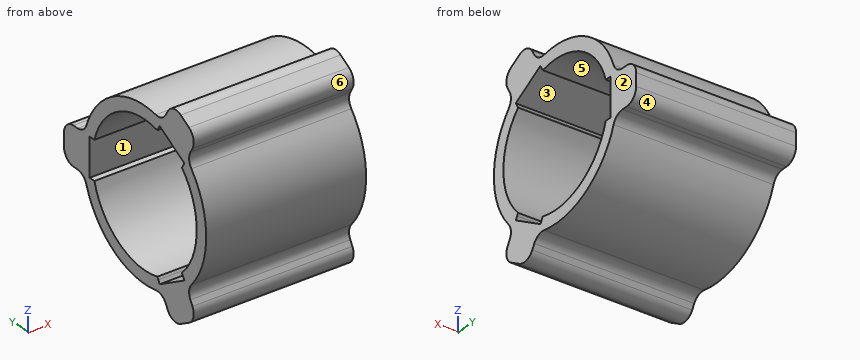
Autodesk Inventor part; units mm, degrees
ref_plane "YZ Plane" through (0, 0, 0) normal (1, 0, 0) x (0, 1, 0)
ref_plane "XZ Plane" through (0, 0, 0) normal (0, 1, 0) x (-1, 0, 0)
ref_plane "XY Plane" through (0, 0, 0) normal (0, 0, 1) x (1, 0, 0)
sketch "Sketch1" plane through (0, 0, 0) normal (1, 0, 0) x (0, 1, 0)
  point P0 (0, 0)
sketch "Sketch2" plane through (0, 0, 0) normal (1, 0, 0) x (0, 1, 0)
  circle A0 centre (0, 0) radius 11
  circle A1 centre (0, 0) radius 13
  line L0 (0, 0) -> (13, 0)
  line L1 (0, 0) -> (-6.5, -11.2583)
  line L2 (0, 0) -> (13, 0) construction
  line L3 (0, 0) -> (-6.5, 11.2583)
  line L4 (0, 0) -> (13, 0) construction
  line L5 (11, 0) -> (11, -3)
  line L6 (11, 0) -> (11, 3)
  line L7 (-5.5, 9.5263) -> (-8.0981, 8.0263)
  line L8 (-5.5, 9.5263) -> (-2.9019, 11.0263)
  line L9 (-5.5, -9.5263) -> (-2.9019, -11.0263)
  line L10 (-5.5, -9.5263) -> (-8.0981, -8.0263)
  line L11 (11, 3) -> (15, 3)
  line L12 (15, 3) -> (11, 3)
  line L13 (11, 3) -> (11, -3)
  line L14 (11, -3) -> (15, -3)
  line L15 (15, -3) -> (15, 3)
  line L16 (-2.9019, 11.0263) -> (-4.9019, 14.4904)
  line L17 (-8.0981, 8.0263) -> (-10.0981, 11.4904)
  line L18 (-10.0981, 11.4904) -> (-4.9019, 14.4904)
  line L19 (-2.9019, -11.0263) -> (-4.9019, -14.4904)
  line L20 (-8.0981, -8.0263) -> (-10.0981, -11.4904)
  line L21 (-4.9019, -14.4904) -> (-10.0981, -11.4904)
  line L22 (-2.9019, 11.0263) -> (-2.6934, 10.6652)
  line L23 (-8.0981, 8.0263) -> (-7.8896, 7.6652)
  line L24 (-2.6934, 10.6652) -> (-3.1934, 11.5312)
  line L25 (-3.1934, 11.5312) -> (-8.3896, 8.5312)
  line L26 (-2.9019, -11.0263) -> (-2.6934, -10.6652)
  line L27 (-8.0981, -8.0263) -> (-7.8896, -7.6652)
  line L28 (-2.6934, -10.6652) -> (-3.1934, -11.5312)
  line L29 (-3.1934, -11.5312) -> (-8.3896, -8.5312)
  line L30 (11, -3) -> (10.583, -3)
  line L31 (11, 3) -> (10.583, 3)
  line L32 (10.583, -3) -> (11.583, -3)
  line L33 (11.583, -3) -> (11.583, 3)
  point P0 (-8.9226, 9.4545)
  point P1 (-8.9226, -9.4545)
  point P2 (-3.7265, -12.4545)
  point P3 (12.6491, -3)
  point P4 (12.6491, 3)
  point P5 (-3.7265, 12.4545)
  dimension "d0" = 22
  dimension "d1" = 26
  dimension "d2" = 120
  dimension "d3" = 120
  dimension "d4" = 3
  dimension "d5" = 3
  dimension "d6" = 3
  dimension "d7" = 3
  dimension "d8" = 3
  dimension "d9" = 3
  dimension "d10" = 4
  dimension "d11" = 4
  dimension "d12" = 4
  dimension "d13" = 4
  dimension "d14" = 4
  dimension "d15" = 1
  dimension "d16" = 1
  dimension "d17" = 1
extrude "Extrusion1" add sketch "Sketch2" along normal blind 25 contours A0 L22 L16 A1 L11 L31 | L30 L14 A1 L19 L26 A0 | L33 L11 A1 L0 | L0 A1 L14 L33 | A1 L11 L15 L14 | L27 L20 A1 L17 L23 A0 | L29 L19 A1 L1 | L1 A1 L20 L29 | L25 L17 A1 L3 | L3 A1 L16 L25 | A1 L19 L21 L20 | A1 L17 L18 L16
sketch "Sketch3" plane through (25, 0, 0) normal (1, 0, 0) x (0, 0, -1)
  line L0 (3, 15) -> (-3, 15)
  line L1 (-3, 15) -> (3, 15)
  line L2 (3, 15) -> (3, 16.9996)
  line L3 (3, 16.9996) -> (-3, 16.9996)
  line L4 (-3, 16.9996) -> (-3, 15)
  line L5 (9.4545, -8.9226) -> (11.4904, -10.0981)
  line L6 (11.4904, -10.0981) -> (13.2224, -11.0981)
  line L7 (13.2224, -11.0981) -> (16.2224, -5.9019)
  line L8 (16.2224, -5.9019) -> (14.4904, -4.9019)
  line L9 (-11.4904, -10.0981) -> (-9.4545, -8.9226)
  line L10 (-11.4904, -10.0981) -> (-13.2224, -11.0981)
  line L11 (-13.2224, -11.0981) -> (-16.2224, -5.9019)
  line L12 (-14.4904, -4.9019) -> (-11.4904, -10.0981)
  line L13 (-16.2224, -5.9019) -> (-14.4904, -4.9019)
  point P0 (0, 0)
  dimension "d20" = 2
  dimension "d21" = 6
  dimension "d22" = 2
  dimension "d23" = 6
extrude "Extrusion2" add sketch "Sketch3" against normal blind 25 contours L0 L4 L3 L2
extrude "Extrusion3" add sketch "Sketch3" against normal blind 25 contours L10 L11 L13 L12
sketch "Sketch4" plane through (0, 0, 0) normal (-1, 0, 0) x (0, 0, 1)
  line L0 (-11.4904, -10.0981) -> (-14.4904, -4.9019)
  line L1 (-11.4904, -10.0981) -> (-14.4904, -4.9019)
  line L2 (-14.4904, -4.9019) -> (-16.2224, -5.9019)
  line L3 (-16.2224, -5.9019) -> (-13.2224, -11.0981)
  line L4 (-13.2224, -11.0981) -> (-11.4904, -10.0981)
  point P0 (0, 0)
  dimension "d28" = 2
  dimension "d29" = 6
extrude "Extrusion4" add sketch "Sketch4" against normal blind 25
fillet "Fillet1" radius 2 12 edges at (12.5, -8.9226, -9.4545) (12.5, -11.0981, -13.2224) (12.5, -3.7265, -12.4545) (12.5, -5.9019, -16.2224) (12.5, 12.6491, -3) (12.5, 16.9996, -3) (12.5, 12.6491, 3) (12.5, 16.9996, 3) (12.5, -3.7265, 12.4545) (12.5, -5.9019, 16.2224) (12.5, -8.9226, 9.4545) (12.5, -11.0981, 13.2224)
properties part number "Part1_3DPrint"
Could you check a few things on this model? Use its own coordinates, in mm. Face numbers are marked on the shaded views. A direction names the side the tool comes from. Coordinates: 2 decimals unless noted, no trailing zeros. Write each loop counter-clockwise with the first axis right and the second up, starting at its lowest first coordinate (ties: lowest second). Pieces come first, ordered by that corner, then holes. Notation, with made-up numbers: (-11.75, 12.5) -> (1.25, 12.5) arc R13 ccw to (1.25, 31.5) -> close; hole circle Ø3 at (-39.5, 9). An arc over 180 degrees is marked (long way). Write item = value, one per line. Start each with the question number.
(1) Will these pins go through, and if not, where does the flat tip stop? pin 1 (3 mm diameter, centred on x = 10, z = 8.5, fed in from +Y); pin 2 (1.5 mm diameter, centred on y = -7.5, z = 4, fed in from -X); pin 3 (2 mm diameter, centred on x = 20.5, z = -9, fed in from -Y); pin 4 (2 mm diameter, centred on x = 20, y = -9.5, fed in from +Z).
(2) We'd pull the mould along Y, two halves only. Please class the marked faces 3, 4, 5 and 6: released by +Y, released by -Y, zero draft, split by the parting line, or undercut.
(3) I need wall thicknesses on line 1 (Z direction, x = 10.75, y = -8); line 2 (Z direction, x = 19.25, y = -10); line 3 (Z direction, x = 1, y = -7). Which ranges of each line are inside material? Lowest first, please. Write a range as [from, to].
(4) Which directions (+Z, -Z, +X, -X, +Y, -Y) give clear straight access to the entire face, cutting with the end or side of a thin tool? Please do the marked faces 1 and 2.
(5) I want a section at B-B (y = -6.25). Please give me the cut outline in (x, z), plus the area to 3 significant figures.
(6) I want a section at A-A (z = 10). Please give me the cut outline in (x, y), plus the area to 3 significant figures.
(7) I want a section at C-C (z = -12). Please give me the cut outline in (x, y).
Result set:
q1.pin_1 = 10.95
q1.pin_2 = through
q1.pin_3 = -10.25
q1.pin_4 = 14.72
q2.face_3 = undercut
q2.face_4 = released by +Y
q2.face_5 = undercut
q2.face_6 = released by -Y
q3.line_1 = [-15.01, -8.76], [-7.86, -7.55], [7.55, 7.86], [8.76, 15.01]
q3.line_2 = [-13.64, -11.32], [-8.31, -4.58], [4.58, 8.31], [11.32, 13.64]
q3.line_3 = [-15.46, -9.33], [9.33, 15.46]
q4.face_1 = +X, -X
q4.face_2 = +Z, -Z, +X, +Y, -Y
q5.outline = (0, -15.45) -> (25, -15.45) -> (25, -9.77) -> (0, -9.77) -> close; (0, 9.77) -> (25, 9.77) -> (25, 15.45) -> (0, 15.45) -> close
q5.area = 284 mm2
q6.outline = (0, -9.42) -> (25, -9.42) -> (25, -5.85) -> (0, -5.85) -> close; (0, 4.58) -> (25, 4.58) -> (25, 8.31) -> (0, 8.31) -> close
q6.area = 182 mm2
q7.outline = (0, -10.31) -> (25, -10.31) -> (25, 5) -> (0, 5) -> close
